from build123d import *

# Parameters (mm, degrees)
F1_DEPTH = 3
F2_R     = 1.5875
F3_DEPTH = 10.901


with BuildPart() as f1:
    # F0 (on Front) → F1 (new body, symmetric)
    with BuildSketch(Plane.XZ):
        with BuildLine():
            Line((-29.1, 18.76), (-29.1, 8.76))
            Line((-29.1, 8.76), (-29.1, -12.24))
            Line((-29.1, -12.24), (-29.1, -22.24))
            ThreePointArc((-29.1, -22.24), (-27.635534, -25.775534), (-24.1, -27.24))
            Line((-24.1, -27.24), (3.4, -27.24))
            ThreePointArc((3.4, -27.24), (5.167767, -27.972233), (5.9, -29.74))
            Line((5.9, -29.74), (5.9, -32.24))
            ThreePointArc((5.9, -32.24), (6.632233, -34.007767), (8.4, -34.74))
            ThreePointArc((8.4, -34.74), (10.167767, -34.007767), (10.9, -32.24))
            Line((10.9, -32.24), (10.9, -30.99))
            Line((10.9, -30.99), (10.9, -27.24))
            Line((10.9, -27.24), (10.9, -12.33))
            ThreePointArc((10.9, -12.33), (0.31, -1.74), (10.9, 8.85))
            Line((10.9, 8.85), (10.9, 23.76))
            Line((10.9, 23.76), (10.9, 27.51))
            Line((10.9, 27.51), (10.9, 28.76))
            ThreePointArc((10.9, 28.76), (10.167767, 30.527767), (8.4, 31.26))
            ThreePointArc((8.4, 31.26), (6.632233, 30.527767), (5.9, 28.76))
            Line((5.9, 28.76), (5.9, 26.26))
            ThreePointArc((5.9, 26.26), (5.167767, 24.492233), (3.4, 23.76))
            Line((3.4, 23.76), (-24.1, 23.76))
            ThreePointArc((-24.1, 23.76), (-27.635534, 22.295534), (-29.1, 18.76))
        make_face()
        with BuildLine():
            ThreePointArc((-20.35, -12.24), (-22.85, -14.74), (-25.35, -12.24))
            ThreePointArc((-25.35, -12.24), (-22.85, -9.74), (-20.35, -12.24))
        make_face(mode=Mode.SUBTRACT)
        with BuildLine():
            ThreePointArc((-11.6, -12.24), (-14.1, -14.74), (-16.6, -12.24))
            ThreePointArc((-16.6, -12.24), (-14.1, -9.74), (-11.6, -12.24))
        make_face(mode=Mode.SUBTRACT)
        with BuildLine():
            ThreePointArc((-25.35, 8.76), (-22.85, 11.26), (-20.35, 8.76))
            ThreePointArc((-20.35, 8.76), (-22.85, 6.26), (-25.35, 8.76))
        make_face(mode=Mode.SUBTRACT)
        with BuildLine():
            ThreePointArc((-11.6, 8.76), (-14.1, 6.26), (-16.6, 8.76))
            ThreePointArc((-16.6, 8.76), (-14.1, 11.26), (-11.6, 8.76))
        make_face(mode=Mode.SUBTRACT)
    extrude(amount=F1_DEPTH, both=True)

    # F2 (on Right) → F3 (cut, through all)
    with BuildSketch(Plane.YZ):
        with Locations((0, 27.51)):
            Circle(F2_R)
        with Locations((0, -30.99)):
            Circle(F2_R)
    extrude(amount=F3_DEPTH, mode=Mode.SUBTRACT)


solid = f1.part
Geometry: final body of the model. Coordinates: model frame, mm. A direction names the side the tool comes from. Coordinates: 2 decimals unless noted, no trailing zeros. Loops run counter-clockwise (first coordinate to the right, second up) from the corner with the lowest first, then second, coordinate; pieces in that order, holes last. Notation, with made-up numbers: M 23,47.5 L 32,47.5 A26 cw 32,86.5 Z; hole C 49,68 d4. An arc over 180 degrees is marked long. One line per item, written item: value. Start each with the question number.
1) Reachability of faces 1 (the flat face through (5.9, 2, 28)), 2 (the cylindrical face through (-20.866, -0.042, -13.761)), 3 (the flat face through (-11, 0, -27.24)) from +Z, -Z, +X, -X, +Y, -Y: full face, straight path, thin tool, end or side. Return the list, or none.
2) Cut plane D-D (z = -0.5). Return loops of the section in (x, y).
3) Cut plane A-A (x = -14.1). Return loops of the section in (y, z), then the cut area to 3 significant figures.
4) Cut plane C-C (z = -30.99). Return loops of the section in (x, y).
5) Draft query along Y for faces 4 (the cylindrical face through (8.35, 0.85, -29.65)), 5 (the flat face through (-9, -3, -1)), 6 (the flat face through (5.9, -2, -31)). Return one class per face: released by +Y, released by -Y, zero draft, split by the parting line, or undercut.
6) Pin query (flat end, axial travel): P1, Ø0.6, axis at y = -1.5, z = -31.5, coming from the -X side; P2, Ø1.8, axis at x = -10, y = -1.5, coming from the -Z side. Return the tip coordinate at first contact, or that it passes through.
7) Cut plane B-B (y = 0). Return loops of the section in (x, z).
8) Material intervals for L1, parallel to Z at x = -14.1, y = -1.05; L2, parallel to X at y = 1.5, z = 8; L3, parallel to X at y = -0.75, z = -10.5, sorted ascending. Write a range as from..to.
Evaluation:
1. face 1: +Z, -X, +Y, -Y
1. face 2: +Y, -Y
1. face 3: -Z, -X, +Y, -Y
2. outline: M -29.1,-3 L 0.38,-3 L 0.38,3 L -29.1,3 Z
3. outline: M -3,-27.24 L 3,-27.24 L 3,-14.74 L -3,-14.74 Z; M -3,-9.74 L 3,-9.74 L 3,6.26 L -3,6.26 Z; M -3,11.26 L 3,11.26 L 3,23.76 L -3,23.76 Z
3. area: 246 mm^2
4. outline: M 5.9,-3 L 10.9,-3 L 10.9,-1.59 L 5.9,-1.59 Z; M 5.9,1.59 L 10.9,1.59 L 10.9,3 L 5.9,3 Z
5. face 4: undercut
5. face 5: released by -Y
5. face 6: zero draft
6. P1: x = 5.9
6. P2: z = -27.24
7. outline: M -29.1,-22.24 A5 ccw -24.1,-27.24 L 3.4,-27.24 A2.5 cw 5.88,-29.4 L 10.9,-29.4 L 10.9,-12.33 A10.59 cw 10.9,8.85 L 10.9,25.92 L 5.88,25.92 A2.5 cw 3.4,23.76 L -24.1,23.76 A5 ccw -29.1,18.76 Z; M 5.92,-32.58 A2.5 ccw 10.88,-32.58 Z; M 5.92,29.1 L 10.88,29.1 A2.5 ccw Z; hole C -22.85,-12.24 d5; hole C -22.85,8.76 d5; hole C -14.1,-12.24 d5; hole C -14.1,8.76 d5
8. L1: -27.24..-14.74, -9.74..6.26, 11.26..23.76
8. L2: -29.1..-25.23, -20.47..-16.48, -11.72..6.74
8. L3: -29.1..-24.65, -21.05..-15.9, -12.3..4.95
